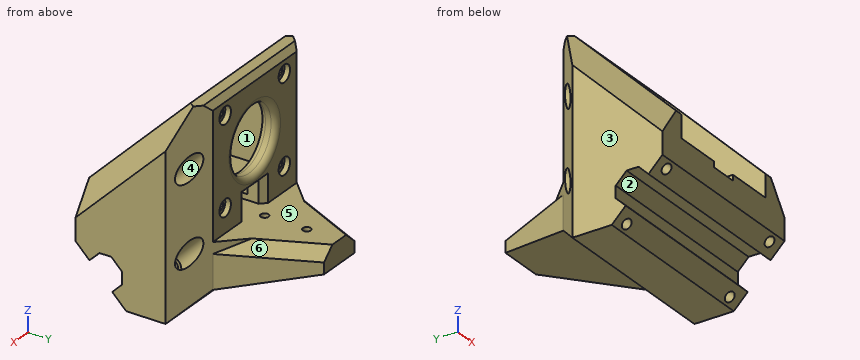
from build123d import *

# Parameters (mm, degrees)
SKETCH1_W           = 28
SKETCH1_H           = 28
BOSS_EXTRUDE1_DEPTH = 64
CHAMFER1_SIZE       = 18
SKETCH3_W           = 64
SKETCH3_H           = 28
BOSS_EXTRUDE2_DEPTH = 14
BOSS_EXTRUDE3_DEPTH = 44
CHAMFER2_SIZE       = 32
SKETCH5_R           = 11.5
SKETCH5_R_2         = 1.8
CUT_EXTRUDE1_DEPTH  = 6
CHAMFER3_SIZE       = 2
SKETCH2_R           = 1.8
CUT_EXTRUDE2_DEPTH  = 96.676538399
SKETCH6_R           = 3
CUT_EXTRUDE3_DEPTH  = 45
SKETCH7_R           = 3
CUT_EXTRUDE4_DEPTH  = 2
FILLET1_R           = 2
CHAMFER4_SIZE       = 10
CHAMFER5_SIZE       = 10
CHAMFER6_START      = -29
CHAMFER6_OUTLINE_W  = 4
CHAMFER6_OUTLINE_H  = 54
CHAMFER6_DEPTH      = 3.544155877
CHAMFER7_SIZE       = 10
SKETCH8_W           = 44
SKETCH8_H           = 16
BOSS_EXTRUDE4_DEPTH = 30
SKETCH9_R           = 1.4
CUT_EXTRUDE5_DEPTH  = 3.5
CHAMFER8_SIZE       = 14
CHAMFER8_SIZE_2     = 30.023096887
CHAMFER9_SIZE       = 8
CHAMFER9_SIZE2      = 29.856406461
CHAMFER10_SIZE      = 4
SKETCH11_W          = 10
SKETCH11_H          = 8
CUT_EXTRUDE6_DEPTH  = 97.041657628
CHAMFER11_SIZE      = 2
SKETCH12_W          = 64
SKETCH12_H          = 11.455844122
CUT_EXTRUDE7_DEPTH  = 8
CHAMFER12_SIZE      = 3


with BuildPart() as part:
    # Sketch1 → Boss-Extrude1 (new body)
    with BuildSketch(Plane(origin=(0, 0, 0), x_dir=(0, 0, -1), z_dir=(1, 0, 0))):
        Rectangle(SKETCH1_W, SKETCH1_H)
    extrude(amount=BOSS_EXTRUDE1_DEPTH)

    # Chamfer1
    chamfer1_edges = [part.edges().sort_by_distance(p)[0] for p in [
        (32, -14, -14),
    ]]
    chamfer(chamfer1_edges, length=CHAMFER1_SIZE)

    # Sketch3 → Boss-Extrude2 (add)
    with BuildSketch(Plane(origin=(0, 14, 0), x_dir=(1, 0, 0), z_dir=(0, 1, 0))):
        with Locations((32, 0)):
            Rectangle(SKETCH3_W, SKETCH3_H)
    extrude(amount=BOSS_EXTRUDE2_DEPTH)

    # Sketch4 → Boss-Extrude3 (add)
    with BuildSketch(Plane.XY.offset(14)):
        Polygon((0, -14), (0, 28), (64, 28), (64, -14), (54, -14), (54, 22), (10, 22), (10, -14), align=None)
    extrude(amount=BOSS_EXTRUDE3_DEPTH)

    # Chamfer2
    chamfer2_edges = [part.edges().sort_by_distance(p)[0] for p in [
        (5, -14, 58),
        (59, -14, 58),
    ]]
    chamfer(chamfer2_edges, length=CHAMFER2_SIZE)

    # Sketch5 → Cut-Extrude1 (cut)
    with BuildSketch(Plane(origin=(0, 22, 0), x_dir=(-1, 0, 0), z_dir=(0, -1, 0))):
        with Locations(Location((-32, -36, 0), (0, 0, 180))):
            Circle(SKETCH5_R)
        with Locations(Location((-16.5, -51.5, 0), (0, 0, 180))):
            Circle(SKETCH5_R_2)
        with Locations(Location((-47.5, -51.5, 0), (0, 0, 180))):
            Circle(SKETCH5_R_2)
        with Locations(Location((-47.5, -20.5, 0), (0, 0, 180))):
            Circle(SKETCH5_R_2)
        with Locations(Location((-16.5, -20.5, 0), (0, 0, 180))):
            Circle(SKETCH5_R_2)
    extrude(amount=-CUT_EXTRUDE1_DEPTH, mode=Mode.SUBTRACT)

    # Chamfer3
    chamfer3_edges = [part.edges().sort_by_distance(p)[0] for p in [
        (32, 28, 58),
    ]]
    chamfer(chamfer3_edges, length=CHAMFER3_SIZE)

    # Sketch2 → Cut-Extrude2 (cut, through all)
    with BuildSketch(Plane(origin=(0, -5, -5), x_dir=(-1, 0, 0), z_dir=(0, -0.7071067811865488, -0.7071067811865464))):
        with Locations(Location((-5, -10, 0), (0, 0, 90))):
            Circle(SKETCH2_R)
        with Locations(Location((-59, -10, 0), (0, 0, 90))):
            Circle(SKETCH2_R)
        with Locations(Location((-59, 10, 0), (0, 0, 90))):
            Circle(SKETCH2_R)
        with Locations(Location((-5, 10, 0), (0, 0, 90))):
            Circle(SKETCH2_R)
    extrude(amount=-CUT_EXTRUDE2_DEPTH, mode=Mode.SUBTRACT)

    # Sketch6 → Cut-Extrude3 (cut)
    with BuildSketch(Plane(origin=(0, 42, 42), x_dir=(1, 0, 0), z_dir=(0, 0.7071067811865477, 0.7071067811865475))):
        with Locations(Location((5, -10, 0), (0, 0, 270))):
            Circle(SKETCH6_R)
        with Locations(Location((5, 10, 0), (0, 0, 270))):
            Circle(SKETCH6_R)
        with Locations(Location((59, 10, 0), (0, 0, 270))):
            Circle(SKETCH6_R)
        with Locations(Location((59, -10, 0), (0, 0, 270))):
            Circle(SKETCH6_R)
    extrude(amount=-CUT_EXTRUDE3_DEPTH, mode=Mode.SUBTRACT)

    # Sketch7 → Cut-Extrude4 (cut)
    with BuildSketch(Plane(origin=(0, 28, 0), x_dir=(1, 0, 0), z_dir=(0, 1, 0))):
        with Locations(Location((16.5, -20.5, 0), (0, 0, 270))):
            Circle(SKETCH7_R)
        with Locations(Location((47.5, -20.5, 0), (0, 0, 270))):
            Circle(SKETCH7_R)
        with Locations(Location((47.5, -51.5, 0), (0, 0, 270))):
            Circle(SKETCH7_R)
        with Locations(Location((16.5, -51.5, 0), (0, 0, 270))):
            Circle(SKETCH7_R)
    extrude(amount=-CUT_EXTRUDE4_DEPTH, mode=Mode.SUBTRACT)

    # Fillet1
    fillet1_edges = [part.edges().sort_by_distance(p)[0] for p in [
        (20.5, 28, 36),
        (20.5, 22, 36),
    ]]
    fillet(fillet1_edges, radius=FILLET1_R)

    # Chamfer4
    # the kernel refuses this chamfer: 10 mm, written as the material it takes off along each edge
    with BuildSketch(Plane(origin=(64, 28, 81.71682988), x_dir=(-1, 0, 0), z_dir=(0, 0, -1))) as chamfer4_piece_1:
        Polygon((CHAMFER4_SIZE, 0), (0, -CHAMFER4_SIZE), (0, 0), align=None)
    extrude(amount=121.433659759, mode=Mode.SUBTRACT)
    with BuildSketch(Plane(origin=(0, 28, 81.71682988), x_dir=(1, 0, 0), z_dir=(0, 0, -1))) as chamfer4_piece_2:
        Polygon((CHAMFER4_SIZE, 0), (0, CHAMFER4_SIZE), (0, 0), align=None)
    extrude(amount=121.433659759, mode=Mode.SUBTRACT)

    # Chamfer5
    chamfer5_edges = [part.edges().sort_by_distance(p)[0] for p in [
        (64, 2, 42),
        (0, 2, 42),
    ]]
    chamfer(chamfer5_edges, length=CHAMFER5_SIZE - 0.0001)  # a hair under: the kernel refuses the full size

    # Chamfer6: read off the stored shape, not the designer's step
    # Chamfer6 outline → Chamfer6 (cut)
    with BuildSketch(Plane(origin=(0, 0, 0), x_dir=(1, 0, 0), z_dir=(0, 0.707106781186549, -0.707106781186546)).offset(CHAMFER6_START)):
        with Locations((8, -31)):
            Rectangle(CHAMFER6_OUTLINE_W, CHAMFER6_OUTLINE_H)
        with Locations((56, -31)):
            Rectangle(CHAMFER6_OUTLINE_W, CHAMFER6_OUTLINE_H)
    extrude(amount=CHAMFER6_DEPTH, mode=Mode.SUBTRACT)

    # Chamfer7
    chamfer7_edges = [part.edges().sort_by_distance(p)[0] for p in [
        (32, 28, -14),
    ]]
    chamfer(chamfer7_edges, length=CHAMFER7_SIZE)

    # Sketch8 → Boss-Extrude4 (add)
    with BuildSketch(Plane(origin=(0, 28, 0), x_dir=(1, 0, 0), z_dir=(0, 1, 0))):
        with Locations((32, -4)):
            Rectangle(SKETCH8_W, SKETCH8_H)
    extrude(amount=BOSS_EXTRUDE4_DEPTH)

    # Sketch9 → Cut-Extrude5 (cut)
    with BuildSketch(Plane.XY.offset(12)):
        with Locations((32, 31.5)):
            Circle(SKETCH9_R)
        with Locations((32, 46.5)):
            Circle(SKETCH9_R)
    extrude(amount=-CUT_EXTRUDE5_DEPTH, mode=Mode.SUBTRACT)

    # Chamfer8
    # the kernel refuses this chamfer: 30.023096887, 14 mm, written as the material it takes off along each edge
    with BuildSketch(Plane(origin=(54, 58, -81.789107611), x_dir=(-1, 0, 0), z_dir=(0, 0, 1))) as chamfer8_piece_1_section:
        Polygon((CHAMFER8_SIZE, 0), (0, CHAMFER8_SIZE_2), (0, 0), align=None)
    chamfer8_piece_1 = extrude(amount=171.578215221, mode=Mode.PRIVATE)
    chamfer8_piece_1 = split(chamfer8_piece_1, bisect_by=Plane(origin=(39, 43, -81.789107611), z_dir=(0.7071067811865476, 0.7071067811865476, 0)), keep=Keep.TOP, mode=Mode.PRIVATE)
    add(chamfer8_piece_1, mode=Mode.SUBTRACT)
    with BuildSketch(Plane(origin=(10, 58, 89.789107611), x_dir=(0, -1, 0), z_dir=(0, 0, -1))) as chamfer8_piece_2_section:
        Polygon((CHAMFER8_SIZE_2, 0), (0, -CHAMFER8_SIZE), (0, 0), align=None)
    chamfer8_piece_2 = extrude(amount=171.578215221, mode=Mode.PRIVATE)
    chamfer8_piece_2 = split(chamfer8_piece_2, bisect_by=Plane(origin=(25, 43, 89.789107611), z_dir=(-0.7071067811865476, 0.7071067811865476, 0)), keep=Keep.TOP, mode=Mode.PRIVATE)
    add(chamfer8_piece_2, mode=Mode.SUBTRACT)

    # Chamfer9
    chamfer9_edges = [part.edges().sort_by_distance(p)[0] for p in [
        (32, 58, -4),
    ]]
    chamfer9_side = [part.faces().sort_by_distance(p)[0] for p in [
        (32, 58, 4),
    ]]
    chamfer(chamfer9_edges, length=CHAMFER9_SIZE, length2=CHAMFER9_SIZE2, reference=chamfer9_side[0])

    # Chamfer10
    chamfer10_edges = [part.edges().sort_by_distance(p)[0] for p in [
        (17.010090322, 43.010090322, 12),
        (46.989909678, 43.010090322, 12),
    ]]
    chamfer(chamfer10_edges, length=CHAMFER10_SIZE)

    # Sketch11 → Cut-Extrude6 (cut, through all)
    with BuildSketch(Plane(origin=(0, 28, 0), x_dir=(1, 0, 0), z_dir=(0, 1, 0))):
        with Locations((32, -16)):
            Rectangle(SKETCH11_W, SKETCH11_H)
    extrude(amount=-CUT_EXTRUDE6_DEPTH, mode=Mode.SUBTRACT)

    # Chamfer11
    chamfer11_edges = [part.edges().sort_by_distance(p)[0] for p in [
        (27, 28, 16),
        (32, 28, 20),
        (37, 28, 16),
    ]]
    chamfer(chamfer11_edges, length=CHAMFER11_SIZE)

    # Sketch12 → Cut-Extrude7 (cut)
    with BuildSketch(Plane(origin=(0, -5, -5), x_dir=(-1, 0, 0), z_dir=(0, -0.7071067811865488, -0.7071067811865464))):
        with Locations((-32, 0)):
            Rectangle(SKETCH12_W, SKETCH12_H)
    extrude(amount=-CUT_EXTRUDE7_DEPTH, mode=Mode.SUBTRACT)

    # Chamfer12
    chamfer12_edges = [part.edges().sort_by_distance(p)[0] for p in [
        (32, -3.393398282, 4.707106781),
        (32, 4.707106781, -3.393398282),
    ]]
    chamfer(chamfer12_edges, length=CHAMFER12_SIZE)


solid = part.part
Check sheet for the modelled part. Datum: model origin and axes. Units: mm. Face numbers are marked on the shaded views. A direction names the side the tool comes from. Round coordinates to 2 decimals unless told otherwise and drop trailing zeros. Write each loop counter-clockwise with the first axis right and the second up, starting at its lowest first coordinate (ties: lowest second). Pieces come first, ordered by that corner, then holes. Notation, with made-up numbers: (9.25, 11) -> (28.25, 11) arc R18 ccw to (28.25, 29) -> close; hole circle Ø4 at (-5, 61.25). An arc over 180 degrees is marked (long way). Answer as CSV lines item,"result". Start each with the question number.
1) Tool access check on the marked faces 1, 2 and 3. Record the directions out of +Z, -Z, +X, -X, +Y, -Y that give a thin tool (end or side, any length) a straight path to the whole face; none if there is none.
2) Section check C-C on x = 16.5. State how many separate pieces and enclosed holes the cut face has, and give its area (3 significant figures).
3) Go/stop test with flat-tipped pins: P1, Ø2, axis at x = 16.5, z = 20.5, coming from the +Y side; P2, Ø4.5, axis at x = 16.5, z = 51.5, coming from the -Y side; P3, Ø3, axis at x = 16.5, z = 50.5, coming from the +Y side; P4, Ø3, axis at y = 10, z = 42.5, coming from the -X side. Record where each tip stops, or that it passes through.
4) Release check for a two-part mould opening along Y. For the marked faces 4, 5 and 6 record: pulls with the +Y half, pulls with the -Y half, needs draft (parallel to the pull), parting line crosses it, or undercut.
5) Section check A-A on z = 51.5. Enter the section's corners in (x, y), and give its area (3 significant figures).
6) Material ranges on line 1 (X direction, y = 5, z = 24.5); line 2 (Z direction, x = 45, y = -10); line 3 (Z direction, x = 16.5, y = 22.9), recorded low to high. Write a range as from..to.
7) Section check B-B on y = 31.5. Enter the section's corners in (x, z), and give its area (3 significant figures).
Found:
1,face 1,"+Z, -Y"
1,face 2,"+X, -X"
1,face 3,"+Z, -Z, -X, +Y, -Y"
2,separate pieces,"3"
2,enclosed holes,"0"
2,area,"1,270 mm^2"
3,P1,"passes through"
3,P2,"stops at y = 22"
3,P3,"stops at y = 26"
3,P4,"stops at x = 3.2"
4,face 4,"undercut"
4,face 5,"needs draft"
4,face 6,"pulls with the +Y half"
5,outline,"(3.17, 21.17) -> (7.17, 15.5) -> (10, 15.5) -> (10, 22) -> (14.7, 22) -> (14.7, 26) -> (13.5, 26) -> (13.5, 28) -> (10, 28) -> close; (18.3, 22) -> (45.7, 22) -> (45.7, 26) -> (44.5, 26) -> (44.5, 28) -> (19.5, 28) -> (19.5, 26) -> (18.3, 26) -> close; (49.3, 22) -> (54, 22) -> (54, 15.5) -> (56.83, 15.5) -> (60.83, 21.17) -> (54, 28) -> (50.5, 28) -> (50.5, 26) -> (49.3, 26) -> close"
5,area,"313 mm^2"
6,line 1,"x = 0..10, 54..64"
6,line 2,"z = 0..14"
6,line 3,"z = -9.1..18.7, 22.3..49.7, 53.3..58"
7,outline,"(11.64, -3.1) -> (52.36, -3.1) -> (52.36, 8) -> (50.5, 9.68) -> (50.5, 12) -> (33.4, 12) -> (33.4, 8.5) -> (30.6, 8.5) -> (30.6, 12) -> (13.5, 12) -> (13.5, 9.68) -> (11.64, 8) -> close"
7,area,"593 mm^2"
